Verification items for the finished model (mm, model axes). Face numbers are marked on the shaded views. A direction names the side the tool comes from. Round coordinates to 2 decimals unless told otherwise and drop trailing zeros. Loops run counter-clockwise (first coordinate to the right, second up) from the corner with the lowest first, then second, coordinate; pieces in that order, holes last. Notation, with made-up numbers: (79, 15) - (93, 15) arc R26 ccw to (93, 51) - close; hole circle Ø8 at (25, 31.5). An arc over 180 degrees is marked (long way). Use a Markdown table: item, result. Add a question column.
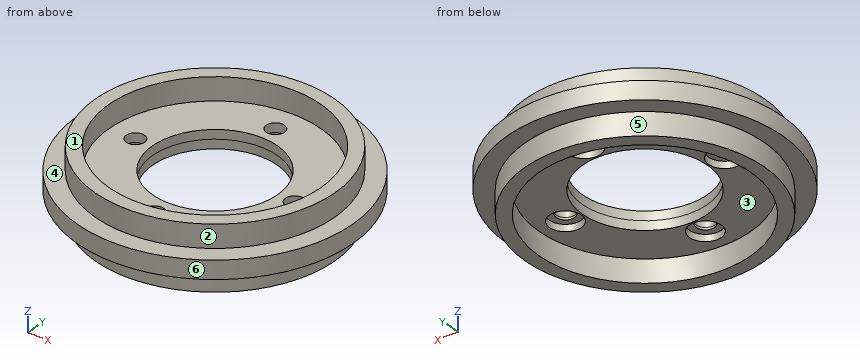
```python
from build123d import *

# Parameters (mm, degrees)
CROQUIS1_R                   = 30.165
CROQUIS1_R_2                 = 13.7
CROQUIS1_R_3                 = 2
SALIENTE_EXTRUIR1_DEPTH      = 2
SALIENTE_EXTRUIR1_DEPTH_BACK = 2
CROQUIS3_R                   = 26.25
CROQUIS3_R_2                 = 23.25
SALIENTE_EXTRUIR2_DEPTH      = 5
CROQUIS4_R                   = 3.5
CORTAR_EXTRUIR1_DEPTH        = 1.5


with BuildPart() as part:
    # Croquis1 → Saliente-Extruir1 (new body, two sides)
    with BuildSketch(Plane.XY) as saliente_extruir1_sk:
        Circle(CROQUIS1_R)
        Circle(CROQUIS1_R_2, mode=Mode.SUBTRACT)
        with Locations((0, 17.5)):
            Circle(CROQUIS1_R_3, mode=Mode.SUBTRACT)
        with Locations((17.5, 0)):
            Circle(CROQUIS1_R_3, mode=Mode.SUBTRACT)
        with Locations((-17.5, 0)):
            Circle(CROQUIS1_R_3, mode=Mode.SUBTRACT)
        with Locations((0, -17.5)):
            Circle(CROQUIS1_R_3, mode=Mode.SUBTRACT)
    extrude(amount=SALIENTE_EXTRUIR1_DEPTH)
    extrude(saliente_extruir1_sk.sketch, amount=-SALIENTE_EXTRUIR1_DEPTH_BACK)

    # Croquis3 → Saliente-Extruir2 (add)
    with BuildSketch(Plane.XY.offset(2)):
        Circle(CROQUIS3_R)
        Circle(CROQUIS3_R_2, mode=Mode.SUBTRACT)
    saliente_extruir2 = extrude(amount=SALIENTE_EXTRUIR2_DEPTH)

    # Croquis4 → Cortar-Extruir1 (cut)
    with BuildSketch(Plane(origin=(0, 0, -2), x_dir=(-1, 0, 0), z_dir=(0, 0, -1))):
        with Locations((0, 17.5)):
            Circle(CROQUIS4_R)
        with Locations((17.5, 0)):
            Circle(CROQUIS4_R)
        with Locations((-17.5, 0)):
            Circle(CROQUIS4_R)
        with Locations((0, -17.5)):
            Circle(CROQUIS4_R)
    extrude(amount=-CORTAR_EXTRUIR1_DEPTH, mode=Mode.SUBTRACT)

    # Simetr_a1: Saliente-Extruir2 across plane
    add(saliente_extruir2.mirror(Plane.XY))


solid = part.part
```
Q1. Release check for a two-part mould opening along Y. For the marked faces 1, 2 and 3 record: +Y half, -Y half, draft (parallel to the pull), parting line (faces both ways), or undercut.
Q2. Set-up check for the marked faces 4, 5 and 6: record each of +Z, -Z, +X, -X, +Y, -Y from which the full face is reachable in a straight line by a thin tool's end or side.
Q3. Section check A-A on x = -17.5. Record the cut outline in (y, z).
Q4. Section check B-B on y = -5. Record the cut outline in (x, z) (3 decimals).
Q5. Thickness scan on line 1 along Y through (x, z) = (0, -0.35) (3 decimals); line 2 along Y through (x, z) = (0, -1.2) (3 decimals); line 3 along Z through (x, y) = (18.5, -21). Record the ranges inside material, lowest first.
Q6. Section check C-C on z = -5. Record the cut outline in (x, y), plus the area to 3 significant figures.
Q7. Section check D-D on x = 0. State how many separate pieces and enclosed holes the cut face has, plus the area to 3 significant figures.
Q8. Go/stop test with flat-tipped pins: pin 1 Ø5 at (x, y) = (5, 13) entering from -Z; pin 2 Ø3.5 at (x, y) = (0.5, -18) entering from -Z; pin 3 Ø6.5 at (x, y) = (0, 17.5) entering from +Z; pin 4 Ø16.5 at (x, y) = (0, 0) entering from +Z. Record where each tip stops, or that it passes through.
Determined:
| question | item | result |
|---|---|---|
| 1 | face 1 | draft |
| 1 | face 2 | parting line |
| 1 | face 3 | undercut |
| 2 | face 4 | +Z |
| 2 | face 5 | -Z |
| 2 | face 6 | +Z, -Z |
| 3 | outline | (-24.57, -2) - (-19.57, -2) - (-19.57, -7) - (-15.31, -7) - (-15.31, -2) - (-3.5, -2) - (-3.5, -0.5) - (-2, -0.5) - (-2, 2) - (-15.31, 2) - (-15.31, 7) - (-19.57, 7) - (-19.57, 2) - (-24.57, 2) - close; (2, -0.5) - (3.5, -0.5) - (3.5, -2) - (15.31, -2) - (15.31, -7) - (19.57, -7) - (19.57, -2) - (24.57, -2) - (24.57, 2) - (19.57, 2) - (19.57, 7) - (15.31, 7) - (15.31, 2) - (2, 2) - close |
| 4 | outline | (-29.748, -2) - (-25.769, -2) - (-25.769, -7) - (-22.706, -7) - (-22.706, -2) - (-12.755, -2) - (-12.755, 2) - (-22.706, 2) - (-22.706, 7) - (-25.769, 7) - (-25.769, 2) - (-29.748, 2) - close; (12.755, -2) - (22.706, -2) - (22.706, -7) - (25.769, -7) - (25.769, -2) - (29.748, -2) - (29.748, 2) - (25.769, 2) - (25.769, 7) - (22.706, 7) - (22.706, 2) - (12.755, 2) - close |
| 5 | line 1 | y = -30.165 to -19.5, -15.5 to -13.7, 13.7 to 15.5, 19.5 to 30.165 |
| 5 | line 2 | y = -30.165 to -21, -14 to -13.7, 13.7 to 14, 21 to 30.165 |
| 5 | line 3 | z = -2 to 2 |
| 6 | outline | circle Ø52.5 at (0, 0); hole circle Ø46.5 at (0, 0) |
| 6 | area | 467 mm² |
| 7 | separate pieces | 4 |
| 7 | enclosed holes | 0 |
| 7 | area | 151 mm² |
| 8 | pin 1 | stops at z = -2 |
| 8 | pin 2 | stops at z = -0.5 |
| 8 | pin 3 | stops at z = 2 |
| 8 | pin 4 | passes through |
